For this review, take the finished solid that the model builds, in its own axes (mm). Face numbers are marked on the shaded views. A direction names the side the tool comes from. Give positions to 0.01 mm unless a question says otherwise; leave off trailing zeros. Write each loop counter-clockwise with the first axis right and the second up, starting at its lowest first coordinate (ties: lowest second). Pieces come first, ordered by that corner, then holes. Notation, with made-up numbers: (-11, 17) -> (43, 17) arc R22 cw to (43, 36) -> close; hole circle Ø3 at (47, -34). An arc over 180 degrees is marked (long way). Return JSON: item names as keys, results as strings.
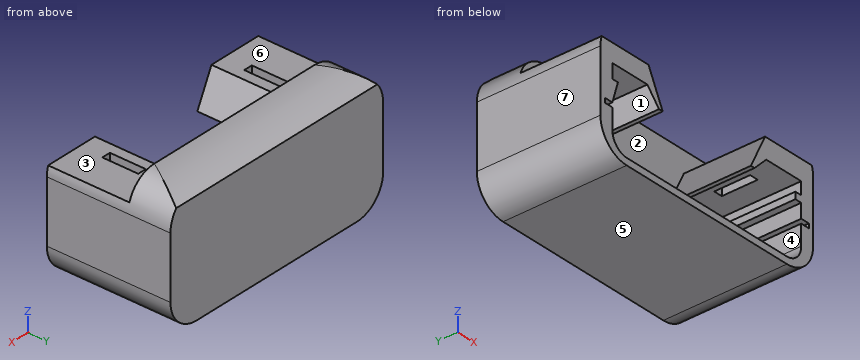
from build123d import *

# Parameters (mm, degrees)
BOX021_W                             = 2.6
BOX021_H                             = 10.6
BOX021_DEPTH                         = 15
BOX020_W                             = 2.6
BOX020_H                             = 10.6
BOX020_DEPTH                         = 15
EXTRUDE056_DEPTH                     = 34.5
EXTRUDE056_ONTO_SKETCH076_ROLL_ANGLE = 90
EXTRUDE055_DEPTH                     = 34.5
EXTRUDE055_ONTO_SKETCH075_ROLL_ANGLE = 90
EXTRUDE057_DEPTH                     = 10.5
EXTRUDE057_ONTO_SKETCH077_ROLL_ANGLE = 90
EXTRUDE060_DEPTH                     = 100
EXTRUDE059_DEPTH                     = 2
EXTRUDE059_ONTO_SKETCH079_ROLL_ANGLE = 90
BOX026_W                             = 80
BOX026_H                             = 28
BOX026_DEPTH                         = 30
EXTRUDE058_DEPTH                     = 35.5
EXTRUDE058_ONTO_SKETCH078_ROLL_ANGLE = 90


with BuildPart() as control_cutout_rec002:
    # Box021 → Box021 (new body)
    with BuildSketch(Plane(origin=(57, 93, 9), x_dir=(1, 0, 0), z_dir=(0, 0, 1))):
        with Locations((1.3, 5.3)):
            Rectangle(BOX021_W, BOX021_H)
    extrude(amount=BOX021_DEPTH)


with BuildPart() as button_cutouts_rec:
    # Box020 → Box020 (new body)
    with BuildSketch(Plane(origin=(8.3, 93, 9), x_dir=(1, 0, 0), z_dir=(0, 0, 1))):
        with Locations((1.3, 5.3)):
            Rectangle(BOX020_W, BOX020_H)
    extrude(amount=BOX020_DEPTH)

    # Fusion034: union control_cutout_rec002
    add(control_cutout_rec002.part)


with BuildPart() as obj1:
    # Sketch076 as drawn → Extrude056 (new)
    with BuildSketch(Plane.XY):
        Polygon((14, 17), (-5.5, 17), (-5.5, 25.6), (73.5, 25.6), (73.5, 17), (54, 17), (49, 6.7), (49, 6.6), (19, 6.6), (19, 6.7), align=None)
    extrude(amount=-EXTRUDE056_DEPTH)


with BuildPart() as obj1_1:
    # Extrude056 onto Sketch076 roll: moved
    add(obj1.part.rotate(Axis((0, 0, 0), (1, 0, 0)), EXTRUDE056_ONTO_SKETCH076_ROLL_ANGLE))


with BuildPart() as obj1_2:
    # Extrude056 onto Sketch076 placement: moved
    add(obj1_1.part.moved(Location((0, 86, 0))))


with BuildPart() as screen_frame001:
    # Sketch075 as drawn → Extrude055 (new)
    with BuildSketch(Plane.XY):
        with BuildLine():
            Line((-2.5, 14.2), (-2.5, 10.6))
            Line((-2.5, 10.6), (1.6, 10.6))
            Line((1.6, 10.6), (1.6, 11.6))
            Line((1.6, 11.6), (13.6, 11.6))
            Line((13.6, 11.6), (17.6, 7))
            Line((17.6, 7), (50.4, 7))
            Line((50.4, 7), (54.4, 11.1))
            Line((54.4, 11.1), (66.4, 11.1))
            Line((66.4, 11.1), (66.4, 10.6))
            Line((66.4, 10.6), (70.5, 10.6))
            Line((70.5, 10.6), (70.5, 14.2))
            ThreePointArc((70.5, 14.2), (67.863961, 20.563961), (61.5, 23.2))
            Line((6.5, 23.2), (61.5, 23.2))
            ThreePointArc((6.5, 23.2), (0.136039, 20.563961), (-2.5, 14.2))
        make_face()
    extrude(amount=-EXTRUDE055_DEPTH)


with BuildPart() as screen_frame001_1:
    # Extrude055 onto Sketch075 roll: moved
    add(screen_frame001.part.rotate(Axis((0, 0, 0), (1, 0, 0)), EXTRUDE055_ONTO_SKETCH075_ROLL_ANGLE))


with BuildPart() as screen_frame001_2:
    # Extrude055 onto Sketch075 placement: moved
    add(screen_frame001_1.part.moved(Location((0, 86, 0))))

    # Cut022: cut obj1
    add(obj1_2.part, mode=Mode.SUBTRACT)


with BuildPart() as cut023:
    # Sketch077 as drawn → Extrude057 (new)
    with BuildSketch(Plane.XY):
        Polygon((13.6, 12.2), (17.6, 7.2), (50.4, 7.2), (54.4, 12.2), align=None)
    extrude(amount=-EXTRUDE057_DEPTH)


with BuildPart() as cut023_1:
    # Extrude057 onto Sketch077 roll: moved
    add(cut023.part.rotate(Axis((0, 0, 0), (1, 0, 0)), EXTRUDE057_ONTO_SKETCH077_ROLL_ANGLE))


with BuildPart() as cut023_2:
    # Extrude057 onto Sketch077 placement: moved
    add(cut023_1.part.moved(Location((0, 110, 0))))

    # Fusion035: union screen_frame001
    add(screen_frame001_2.part)

    # Cut023: cut button_cutouts_rec
    add(button_cutouts_rec.part, mode=Mode.SUBTRACT)


with BuildPart() as round_cut001:
    # Sketch080 → Extrude060 (new body)
    with BuildSketch(Plane.YZ.offset(-14)):
        with BuildLine():
            Line((100, 23.2), (100, 26.2))
            Line((100, 26.2), (138, 26.2))
            Line((138, 26.2), (138, -11.8))
            Line((138, -11.8), (135, -11.8))
            Line((135, -11.8), (135, -1.8))
            ThreePointArc((135, -1.8), (127.67767, 15.87767), (110, 23.2))
            Line((100, 23.2), (110, 23.2))
        make_face()
    extrude(amount=EXTRUDE060_DEPTH)


with BuildPart() as extrude059:
    # Sketch079 as drawn → Extrude059 (new)
    with BuildSketch(Plane.XY):
        with BuildLine():
            Line((-2.5, 14.2), (-2.5, -4.1))
            ThreePointArc((-2.5, -4.1), (0.136039, -10.463961), (6.5, -13.1))
            Line((6.5, -13.1), (61.5, -13.1))
            ThreePointArc((61.5, -13.1), (67.863961, -10.463961), (70.5, -4.1))
            Line((70.5, -4.1), (70.5, 14.2))
            ThreePointArc((70.5, 14.2), (67.863961, 20.563961), (61.5, 23.2))
            Line((6.5, 23.2), (61.5, 23.2))
            ThreePointArc((6.5, 23.2), (0.136039, 20.563961), (-2.5, 14.2))
        make_face()
    extrude(amount=-EXTRUDE059_DEPTH)


with BuildPart() as extrude059_1:
    # Extrude059 onto Sketch079 roll: moved
    add(extrude059.part.rotate(Axis((0, 0, 0), (1, 0, 0)), EXTRUDE059_ONTO_SKETCH079_ROLL_ANGLE))


with BuildPart() as extrude059_2:
    # Extrude059 onto Sketch079 placement: moved
    add(extrude059_1.part.moved(Location((0, 120, 0))))


with BuildPart() as extrude059_3:
    # Extrude059 placement: moved
    add(extrude059_2.part.moved(Location((0, 0.5, 0))))


with BuildPart() as cube007:
    # Box026 → Box026 (new body)
    with BuildSketch(Plane(origin=(-5, 82, 10.6), x_dir=(1, 0, 0), z_dir=(0, 0, 1))):
        with Locations((40, 14)):
            Rectangle(BOX026_W, BOX026_H)
    extrude(amount=BOX026_DEPTH)


with BuildPart() as shell_upper:
    # Sketch078 as drawn → Extrude058 (new)
    with BuildSketch(Plane.XY):
        with BuildLine():
            Line((-2.5, 14.2), (-2.5, -4.1))
            ThreePointArc((-2.5, -4.1), (0.136039, -10.463961), (6.5, -13.1))
            Line((6.5, -13.1), (61.5, -13.1))
            ThreePointArc((61.5, -13.1), (67.863961, -10.463961), (70.5, -4.1))
            Line((70.5, -4.1), (70.5, 14.2))
            ThreePointArc((70.5, 14.2), (67.863961, 20.563961), (61.5, 23.2))
            Line((6.5, 23.2), (61.5, 23.2))
            ThreePointArc((6.5, 23.2), (0.136039, 20.563961), (-2.5, 14.2))
        make_face()
        with BuildLine():
            Line((1.6, 1.2), (-1, 1.2))
            Line((-1, 1.2), (-1, -0.1))
            Line((-1, -0.1), (1.6, -0.1))
            Line((1.6, -0.1), (1.6, -6.1))
            ThreePointArc((1.6, -6.1), (3.064466, -9.635534), (6.6, -11.1))
            Line((6.6, -11.1), (61.4, -11.1))
            ThreePointArc((61.4, -11.1), (64.935534, -9.635534), (66.4, -6.1))
            Line((66.4, -0.1), (66.4, -6.1))
            Line((69, -0.1), (66.4, -0.1))
            Line((69, 1.2), (69, -0.1))
            Line((66.4, 1.2), (69, 1.2))
            Line((66.4, 5.4), (66.4, 1.2))
            Line((64.4, 5.4), (66.4, 5.4))
            Line((64.4, 7.4), (64.4, 5.4))
            Line((66.4, 7.4), (64.4, 7.4))
            Line((66.4, 10.6), (66.4, 7.4))
            Line((66.4, 10.6), (66.4, 10.8))
            Line((66.4, 10.8), (64.5, 10.8))
            Line((64.5, 10.8), (3.5, 10.8))
            Line((1.6, 10.8), (3.5, 10.8))
            Line((1.6, 10.6), (1.6, 10.8))
            Line((1.6, 10.6), (1.6, 7.4))
            Line((1.6, 7.4), (3.5, 7.4))
            Line((3.5, 7.4), (1.6, 1.2))
        make_face(mode=Mode.SUBTRACT)
    extrude(amount=EXTRUDE058_DEPTH)


with BuildPart() as shell_upper_1:
    # Extrude058 onto Sketch078 roll: moved
    add(shell_upper.part.rotate(Axis((0, 0, 0), (1, 0, 0)), EXTRUDE058_ONTO_SKETCH078_ROLL_ANGLE))


with BuildPart() as shell_upper_2:
    # Extrude058 onto Sketch078 placement: moved
    add(shell_upper_1.part.moved(Location((0, 120, 0))))


with BuildPart() as shell_upper_3:
    # Extrude058 placement: moved
    add(shell_upper_2.part.moved(Location((0, 1.5, 0))))

    # Cut024: cut Cube007
    add(cube007.part, mode=Mode.SUBTRACT)

    # Fusion038: union Extrude059
    add(extrude059_3.part)

    # Cut025: cut round_cut001
    add(round_cut001.part, mode=Mode.SUBTRACT)

    # Fusion039: union Cut023
    add(cut023_2.part)


solid = shell_upper_3.part
1. Add section B-B, the plane x = 20. State the section outline as (y, z) points, plus the area to 3 significant figures.
Results found:
{"outline": "(86, -13.1) -> (122.5, -13.1) -> (122.5, 19.85) arc R25 ccw to (110, 23.2) -> (110, 7.2) -> (120.5, 7.2) -> (120.5, -11.1) -> (86, -11.1) -> close", "area": "296 mm²"}
2. For pin 1 (3 mm diameter, centred on x = 18, z = 15, fed in from -Y); pin 2 (12 mm diameter, centred on x = 57, y = 103.5, fed in from +Z); pin 3 (3 mm diameter, centred on x = 0.5, y = 102, fed in from -Z), all flat-tipped, find the tip position at first contact; note any pin that passes through.
Results found:
{"pin 1": "stops at y = 110", "pin 2": "stops at z = 17", "pin 3": "stops at z = -11.89"}
3. Add section D-D, the plane x = 58. State the section outline as (y, z) points, plus the area to 3 significant figures.
Results found:
{"outline": "(86, -13.1) -> (122.5, -13.1) -> (122.5, 19.85) arc R25 ccw to (110, 23.2) -> (110, 17) -> (103.6, 17) -> (103.6, 11.1) -> (110, 11.1) -> (110, 10.8) -> (120.5, 10.8) -> (120.5, -11.1) -> (86, -11.1) -> close; (86, 11.1) -> (93, 11.1) -> (93, 17) -> (86, 17) -> close", "area": "337 mm²"}
4. Add section A-A, the plane x = 9.5. State the section outline as (y, z) points.
Results found:
{"outline": "(86, -13.1) -> (122.5, -13.1) -> (122.5, 19.85) arc R25 ccw to (110, 23.2) -> (110, 17) -> (103.6, 17) -> (103.6, 11.6) -> (110, 11.6) -> (110, 10.8) -> (120.5, 10.8) -> (120.5, -11.1) -> (86, -11.1) -> close; (86, 11.6) -> (93, 11.6) -> (93, 17) -> (86, 17) -> close"}
5. For the marked faces 1, 2 and 3, list the 3-axis set-ups (+Z, -Z, +X, -X, +Y, -Y) from which the entire face can be reached by the end or side of a thin tool; tool diameter is ignored.
Results found:
{"face 1": "-Y", "face 2": "+Z, -Y", "face 3": "+Z, +X, -X, -Y"}
6. Add section C-C, the plane z = 15.5. State the section outline as (x, y) points, plus the area to 3 significant figures.
Results found:
{"outline": "(-2.41, 86) -> (14.73, 86) -> (14.73, 110) -> (53.27, 110) -> (53.27, 86) -> (70.41, 86) -> (70.41, 122.5) -> (-2.41, 122.5) -> close; hole (8.3, 93) -> (10.9, 93) -> (10.9, 103.6) -> (8.3, 103.6) -> close; hole (57, 93) -> (59.6, 93) -> (59.6, 103.6) -> (57, 103.6) -> close", "area": "1,680 mm²"}
7. The part is to be moulded in two halves that separate along Z. For the marked faces 4, 5, 6 and 7, say which applies: +Z half, -Z half, draft (parallel to the pull), parting line (faces both ways), or undercut.
Results found:
{"face 4": "undercut", "face 5": "-Z half", "face 6": "+Z half", "face 7": "draft"}
8. To check wall thickness, follow probe 1 along Y at (x, z) = (10.5, 16); probe 2 along Z at (x, y) = (13.5, 104.5); probe 3 along X at (y, z) = (108, -3). State the ranges of each line that lie inside material, in increasing order.
Results found:
{"probe 1": "y = 86 to 93, 103.6 to 122.5", "probe 2": "z = -13.1 to -11.1, 11.6 to 17", "probe 3": "x = -2.5 to 1.6, 66.4 to 70.5"}
